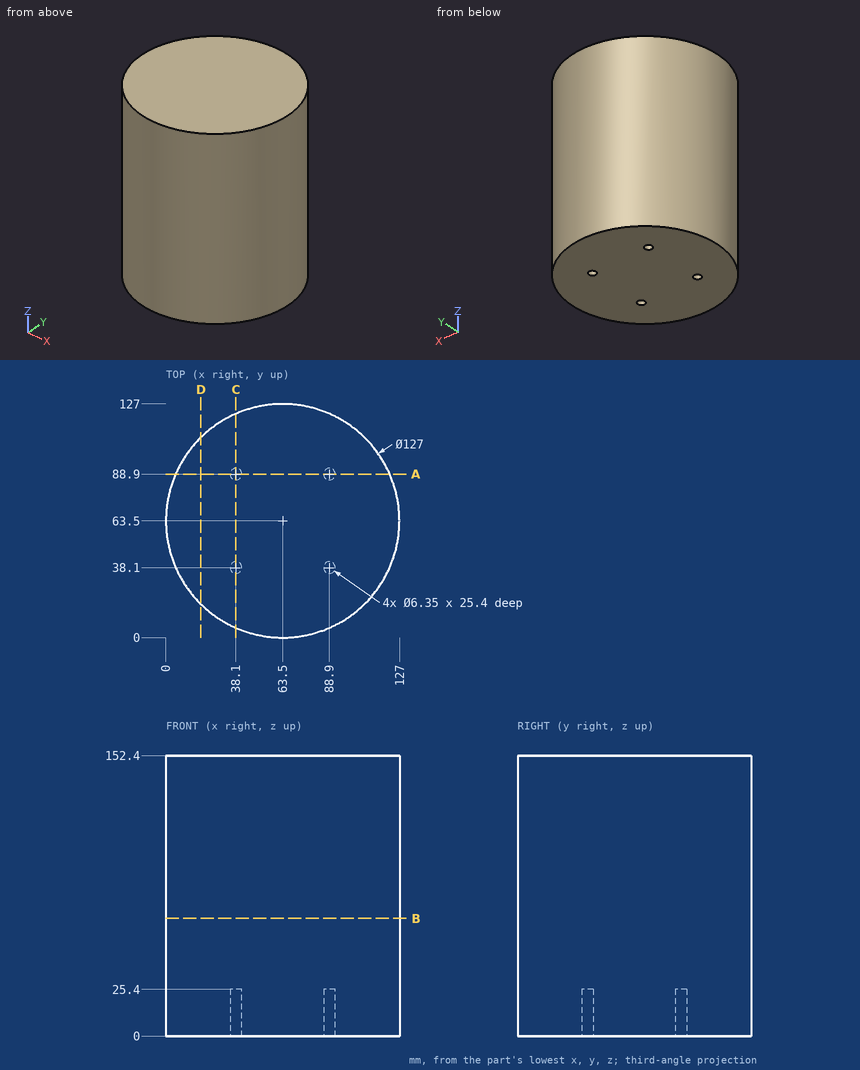
Print and shaded views of the part. All mm, measured from the part's lowest x, y and z. Give positions to 0.01 mm unless a question says otherwise; leave off trailing zeros. Loops run counter-clockwise (first coordinate to the right, second up) from the corner with the lowest first, then second, coordinate; pieces in that order, holes last. Notation, with made-up numbers: (85, -20) -> (141, -20) arc R28 ccw to (141, -2) -> close; hole circle Ø3 at (45, 78.5). An arc over 180 degrees is marked (long way). Use a Markdown table: item, result.
1. Flat gauge pins, fed straight in: pin 1 (5 mm diameter, centred on x = 89, y = 88.5, fed in from -Z); pin 2 (1 mm diameter, centred on y = 52.5, z = 76, fed in from +X); pin 3 (2 mm diameter, centred on y = 87.5, z = 84.5, fed in from -X). Where does each tip first touch, or does it go through?
Check result:
| item | result |
|---|---|
| pin 1 | stops at z = 25.4 |
| pin 2 | stops at x = 126.13 |
| pin 3 | stops at x = 4.31 |
2. Slice it at A-A (y = 88.9). List the corners of the cut face in (x, z) (3 decimals), plus the area to 3 significant figures.
Check result:
| item | result |
|---|---|
| outline | (5.301, 0) -> (34.925, 0) -> (34.925, 25.4) -> (41.275, 25.4) -> (41.275, 0) -> (85.725, 0) -> (85.725, 25.4) -> (92.075, 25.4) -> (92.075, 0) -> (121.699, 0) -> (121.699, 152.4) -> (5.301, 152.4) -> close |
| area | 17,400 mm^2 |
3. Wall check: L1, parallel to Y at x = 38.1, z = 11.5 (3 decimals); L2, parallel to Y at x = 38, z = 18; L3, parallel to X at y = 88, z = 9. Give the ranges that are in metal, low to high. Write a range as [from, to].
Check result:
| item | result |
|---|---|
| L1 | y = [5.301, 34.925], [41.275, 85.725], [92.075, 121.699] |
| L2 | y = [5.35, 34.93], [41.27, 85.73], [92.07, 121.65] |
| L3 | x = [4.92, 35.06], [41.14, 85.86], [91.94, 122.08] |
4. Slice it at B-B (z = 64). List the corners of the cut face in (x, y).
Check result:
| item | result |
|---|---|
| outline | circle Ø127 at (63.5, 63.5) |
5. Slice it at D-D (x = 19). List the corners of the cut face in (y, z).
Check result:
| item | result |
|---|---|
| outline | (18.2, 0) -> (108.8, 0) -> (108.8, 152.4) -> (18.2, 152.4) -> close |
